Read the model definition and answer for the solid it produces. Units are mm, in the model's axes. A direction names the side the tool comes from. Coordinates: 2 decimals unless noted, no trailing zeros. Order: outer loops, then holes, each group sorted by start corner. A loop starts at its lowest first (then second) coordinate and runs counter-clockwise, first axis right, second up.
```python
from build123d import *

# Parameters (mm, degrees)
BOSS_EXTRUDE1_DEPTH = 2.54
BOSS_EXTRUDE2_DEPTH = 12.7
SKETCH3_R           = 1.5875
CUT_EXTRUDE1_DEPTH  = 5.08
CUT_EXTRUDE2_DEPTH  = 1.27


with BuildPart() as part:
    # Sketch1 → Boss-Extrude1 (new body)
    with BuildSketch(Plane.XY):
        with BuildLine():
            Line((33.02, -15.24), (-33.02, -15.24))
            ThreePointArc((-33.02, -15.24), (-34.816051224, -14.496051224), (-35.56, -12.7))
            Line((-35.56, -12.7), (-35.56, 12.7))
            ThreePointArc((-35.56, 12.7), (-34.816051224, 14.496051224), (-33.02, 15.24))
            Line((-33.02, 15.24), (33.02, 15.24))
            ThreePointArc((33.02, 15.24), (34.816051224, 14.496051224), (35.56, 12.7))
            Line((35.56, 12.7), (35.56, -12.7))
            ThreePointArc((35.56, -12.7), (34.816051224, -14.496051224), (33.02, -15.24))
        make_face()
    extrude(amount=BOSS_EXTRUDE1_DEPTH)

    # Sketch2 → Boss-Extrude2 (add)
    with BuildSketch(Plane(origin=(0, 0, 0), x_dir=(-1, 0, 0), z_dir=(0, 0, -1))):
        with BuildLine():
            Line((-34.831192975, 3.429443631), (-34.831192975, -3.429443631))
            ThreePointArc((-34.831192975, -3.429443631), (-34.459218588, -4.327469243), (-33.561192975, -4.699443631))
            Line((-33.561192975, -4.699443631), (-30.365638197, -4.699443631))
            ThreePointArc((-30.365638197, -4.699443631), (-28.120574167, -5.629379601), (-27.190638197, -7.874443631))
            Line((-27.190638197, -7.874443631), (-27.190638197, -13.426949666))
            ThreePointArc((-27.190638197, -13.426949666), (-26.818663809, -14.324975278), (-25.920638197, -14.696949666))
            Line((-25.920638197, -14.696949666), (24.081493188, -14.696949666))
            ThreePointArc((24.081493188, -14.696949666), (24.9795188, -14.324975278), (25.351493188, -13.426949666))
            Line((25.351493188, -13.426949666), (25.351493188, -7.874443631))
            ThreePointArc((25.351493188, -7.874443631), (26.281429158, -5.629379601), (28.526493188, -4.699443631))
            Line((28.526493188, -4.699443631), (31.722047967, -4.699443631))
            ThreePointArc((31.722047967, -4.699443631), (32.620073579, -4.327469243), (32.992047967, -3.429443631))
            Line((32.992047967, -3.429443631), (32.992047967, 3.429443631))
            ThreePointArc((32.992047967, 3.429443631), (32.620073579, 4.327469243), (31.722047967, 4.699443631))
            Line((31.722047967, 4.699443631), (28.526493188, 4.699443631))
            ThreePointArc((28.526493188, 4.699443631), (26.281429158, 5.629379601), (25.351493188, 7.874443631))
            Line((25.351493188, 7.874443631), (25.351493188, 13.426949666))
            ThreePointArc((25.351493188, 13.426949666), (24.9795188, 14.324975278), (24.081493188, 14.696949666))
            Line((24.081493188, 14.696949666), (-25.920638197, 14.696949666))
            ThreePointArc((-25.920638197, 14.696949666), (-26.818663809, 14.324975278), (-27.190638197, 13.426949666))
            Line((-27.190638197, 13.426949666), (-27.190638197, 7.874443631))
            ThreePointArc((-27.190638197, 7.874443631), (-28.120574167, 5.629379601), (-30.365638197, 4.699443631))
            Line((-30.365638197, 4.699443631), (-33.561192975, 4.699443631))
            ThreePointArc((-33.561192975, 4.699443631), (-34.459218588, 4.327469243), (-34.831192975, 3.429443631))
        make_face()
    extrude(amount=BOSS_EXTRUDE2_DEPTH)

    # Sketch3 → Cut-Extrude1 (cut)
    with BuildSketch(Plane.XY.offset(2.54)):
        with Locations((32.7025, -12.065)):
            Circle(SKETCH3_R)
        with Locations((32.7025, 12.065)):
            Circle(SKETCH3_R)
        with Locations((-32.7025, 12.065)):
            Circle(SKETCH3_R)
        with Locations((-32.7025, -12.065)):
            Circle(SKETCH3_R)
    extrude(amount=-CUT_EXTRUDE1_DEPTH, mode=Mode.SUBTRACT)

    # Sketch4 → Cut-Extrude2 (cut)
    with BuildSketch(Plane.XY.offset(2.54)):
        with BuildLine():
            Line((-35.56, -6.017135468), (-29.319201094, -6.017135468))
            ThreePointArc((-29.319201094, -6.017135468), (-27.074137064, -6.947071437), (-26.144201094, -9.192135468))
            Line((-26.144201094, -9.192135468), (-26.144201094, -15.24))
            Line((-26.144201094, -15.24), (-35.56, -15.24))
            Line((-35.56, -15.24), (-35.56, -6.017135468))
        make_face()
        with BuildLine():
            Line((35.56, -6.017135468), (29.50710146, -6.017135468))
            ThreePointArc((29.50710146, -6.017135468), (27.26203743, -6.947071437), (26.33210146, -9.192135468))
            Line((26.33210146, -9.192135468), (26.33210146, -15.24))
            Line((26.33210146, -15.24), (35.56, -15.24))
            Line((35.56, -15.24), (35.56, -6.017135468))
        make_face()
        with BuildLine():
            Line((26.33210146, 9.192135468), (26.33210146, 15.24))
            Line((26.33210146, 15.24), (35.56, 15.24))
            Line((35.56, 15.24), (35.56, 6.017135468))
            Line((35.56, 6.017135468), (29.50710146, 6.017135468))
            ThreePointArc((29.50710146, 6.017135468), (27.26203743, 6.947071437), (26.33210146, 9.192135468))
        make_face()
        with BuildLine():
            Line((-26.144201094, 9.192135468), (-26.144201094, 15.24))
            Line((-26.144201094, 15.24), (-35.56, 15.24))
            Line((-35.56, 15.24), (-35.56, 6.017135468))
            Line((-35.56, 6.017135468), (-29.319201094, 6.017135468))
            ThreePointArc((-29.319201094, 6.017135468), (-27.074137064, 6.947071437), (-26.144201094, 9.192135468))
        make_face()
    extrude(amount=-CUT_EXTRUDE2_DEPTH, mode=Mode.SUBTRACT)


solid = part.part
```
1) A cutting plane is placed at A-A, the plane x = -9.5. Determine the outline of the cut face in (y, z), and give its area (3 significant figures).
A:
outline: (-15.24, 0) - (-14.7, 0) - (-14.7, -12.7) - (14.7, -12.7) - (14.7, 0) - (15.24, 0) - (15.24, 2.54) - (-15.24, 2.54) - close
area: 451 mm2
2) Flat-ended cylindrical pins translate along their axes: pin 1 Ø2 at (y, z) = (-1, -7.5) entering from -X; pin 2 Ø4.5 at (x, y) = (-31, 9) entering from +Z; pin 3 Ø1.5 at (y, z) = (11.5, -8) entering from +X; pin 4 Ø1.9 at (x, y) = (32.7, 12.06) entering from -Z. Find the tip coordinate at first contact, or state that the pin passes through.
A:
pin 1: stops at x = -32.99
pin 2: stops at z = 1.27
pin 3: stops at x = 27.19
pin 4: passes through
3) Straight lines are drawn through the part: line 1 (Y direction, x = 14, z = -6.75); line 2 (Z direction, x = -26.5, y = 8); line 3 (X direction, y = 8.5, z = -10.5). For each, find the intervals that lie inside material, in ascending order.
A:
line 1: y = -14.7 to 14.7
line 2: z = 0 to 1.27
line 3: x = -25.35 to 27.19
4) Determine the mould class of faces 1 (the cylindrical face through (-31.849, -10.726, 0.644)), 2 (the cylindrical face through (28.15, -5.6, -6.26)), 3 (the flat face through (33, 6.017, 2)) for opening direction Y: pulls with the +Y half, pulls with the -Y half, needs draft (parallel to the pull), parting line crosses it, or undercut.
A:
face 1: undercut
face 2: pulls with the -Y half
face 3: pulls with the +Y half
5) A cutting plane is placed at C-C, the plane y = -2.5. Determine the outline of the cut face in (x, z).
A:
outline: (-35.56, 0) - (-32.99, 0) - (-32.99, -12.7) - (34.83, -12.7) - (34.83, 0) - (35.56, 0) - (35.56, 2.54) - (-35.56, 2.54) - close
6) A cutting plane is placed at D-D, the plane y = 7. Determine the outline of the cut face in (x, z), and give its area (3 significant figures).
A:
outline: (-35.56, 0) - (-25.47, 0) - (-25.47, -12.7) - (27.31, -12.7) - (27.31, 0) - (35.56, 0) - (35.56, 1.27) - (27.21, 1.27) - (27.21, 2.54) - (-27.02, 2.54) - (-27.02, 1.27) - (-35.56, 1.27) - close
area: 830 mm2
7) Which of the six approach directions +Z, -Z, +X, -X, +Y, -Y give full straight-line access (tool end or side, diameter ignored) to faces 4 (the cylindrical face through (34.469, -4.318, -6.261)), 5 (the cylindrical face through (-27.1, -6.92, 1.91)), 6 (the flat face through (-31, 11, 1.27))?
A:
face 4: -Z, +X, -Y
face 5: +Z, -X, -Y
face 6: +Z, -X, +Y
